Input: dimensioned drawing with shaded views. Units: mm. Origin: part minimum x, y, z. Round coordinates to 2 decimals unless told otherwise and drop trailing zeros. Order: outer loops, then holes, each group sorted by start corner. A loop starts at its lowest first (then second) coordinate and runs counter-clockwise, first axis right, second up. Notation, with made-up numbers: (20.25, -6) - (55.25, -6) arc R19 ccw to (55.25, 22) - close; hole circle Ø5 at (-12, 57). An arc over 180 degrees is marked (long way). One line per item, written item: value. Start each with the question number.
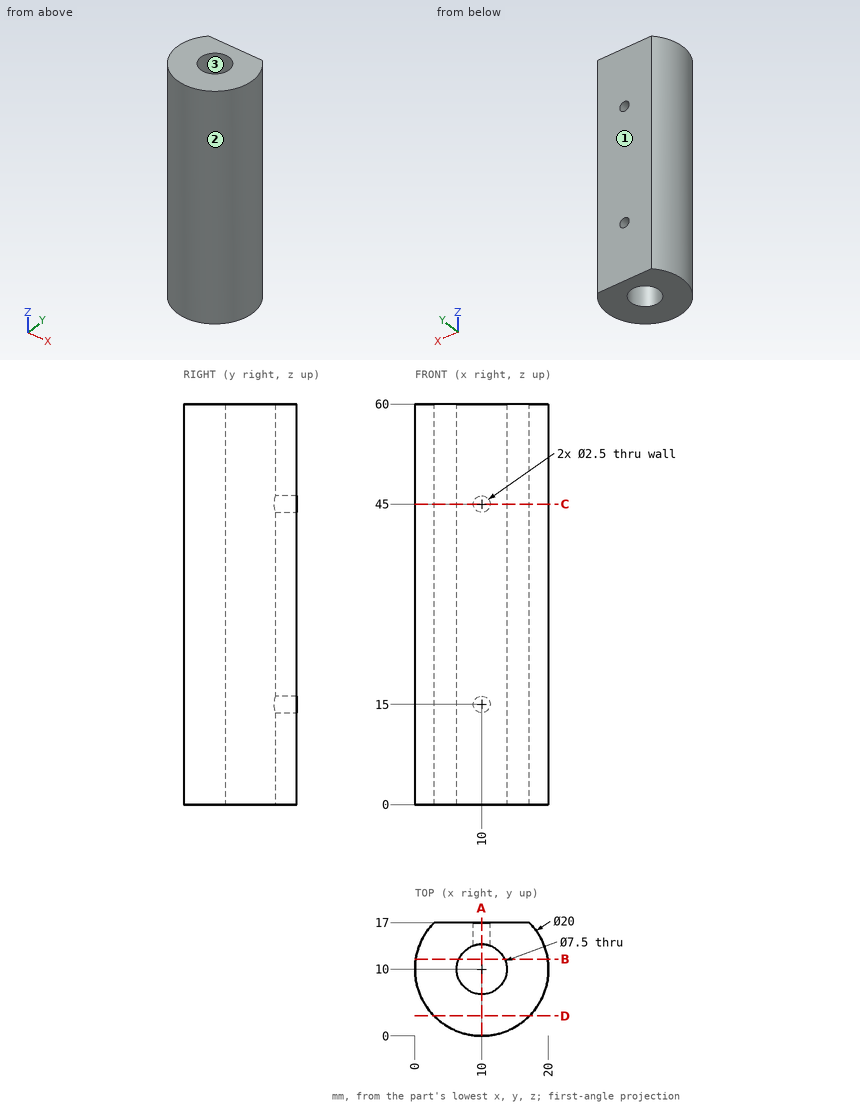
1. Section C-C (z = 45). Return the cut outline in (x, y), then the cut area to 3 significant figures.
2. Pull-direction query (X, two-part tool) for the marked faces 1, 2 and 3; classes: released by +X, released by -X, zero draft, split by the parting line, or undercut.
3. Section A-A (x = 10). Return the cut outline in (y, z).
4. Section B-B (y = 11.5). Return the cut outline in (x, z), then the cut area to 3 significant figures.
5. Pin query (flat end, axial travel): pin 1 (1.5 mm diameter, centred on x = 5, z = 32.5, fed in from -Y); pin 2 (5 mm diameter, centred on y = 8.5, z = 41.5, fed in from -X); pin 3 (4 mm diameter, centred on y = 13.5, z = 7.5, fed in from +X); pin 4 (8 mm diameter, centred on y = 2, z = 19.5, fed in from +X). Return the tip coordinate at first contact, or that it passes through.
6. Section D-D (y = 3). Return the cut outline in (x, z), then the cut area to 3 significant figures.
7. Line query: line 1 (X direction, y = 13.25, z = 22.5); line 2 (X direction, y = 15.8, z = 15); line 3 (Y direction, x = 11.75, z = 21). Output: solid intervals per line, ascending. Write a range as from..to.
Solved:
1. outline: (2.86, 17) arc R10 ccw (long way) to (17.14, 17) - (11.25, 17) - (11.25, 13.54) arc R3.75 cw (long way) to (8.75, 13.54) - (8.75, 17) - close
1. area: 232 mm²
2. face 1: zero draft
2. face 2: split by the parting line
2. face 3: undercut
3. outline: (0, 0) - (6.25, 0) - (6.25, 60) - (0, 60) - close; (13.75, 0) - (17, 0) - (17, 13.75) - (13.75, 13.75) - close; (13.75, 16.25) - (17, 16.25) - (17, 43.75) - (13.75, 43.75) - close; (13.75, 46.25) - (17, 46.25) - (17, 60) - (13.75, 60) - close
4. outline: (0.11, 0) - (6.56, 0) - (6.56, 60) - (0.11, 60) - close; (13.44, 0) - (19.89, 0) - (19.89, 60) - (13.44, 60) - close
4. area: 774 mm²
5. pin 1: stops at y = 0.95
5. pin 2: stops at x = 0
5. pin 3: stops at x = 19.89
5. pin 4: stops at x = 19.17
6. outline: (2.86, 0) - (17.14, 0) - (17.14, 60) - (2.86, 60) - close
6. area: 857 mm²
7. line 1: x = 0.54..8.13, 11.87..19.46
7. line 2: x = 1.85..8.75, 11.25..18.15
7. line 3: y = 0.15..6.68, 13.32..17
